```python
from build123d import *

# Parameters (mm, degrees)
BOSS_EXTRUDE1_DEPTH = 10
CUT_SWEEP1_START    = 7
CUT_SWEEP1_DEPTH    = 3


# Read off the part's stored shape, not the designer's step: Cut-Sweep1
with BuildPart() as part:
    # Sketch1 → Boss-Extrude1 (new body)
    with BuildSketch(Plane(origin=(0, 0, 0), x_dir=(1, 0, 0), z_dir=(0, 1, 0))):
        with BuildLine():
            Line((-35, 0), (35, 0))
            Line((35, 0), (35, 50))
            ThreePointArc((35, 50), (150, 165), (265, 50))
            Line((265, 50), (265, 0))
            Line((265, 0), (335, 0))
            Line((335, 0), (335, 50))
            ThreePointArc((335, 50), (150, 235), (-35, 50))
            Line((-35, 50), (-35, 0))
        make_face()
    extrude(amount=BOSS_EXTRUDE1_DEPTH)

    # Cut-Sweep1 outline → Cut-Sweep1 (cut)
    with BuildSketch(Plane(origin=(0, 0, 0), x_dir=(1, 0, 0), z_dir=(0, 1, 0)).offset(CUT_SWEEP1_START)):
        with BuildLine():
            Line((-30, 50), (-30, 0))
            Line((-30, 0), (-20, 0))
            Line((-20, 0), (-20, 50))
            ThreePointArc((-20, 50), (150, 220), (320, 50))
            Line((320, 50), (320, 0))
            Line((320, 0), (330, 0))
            Line((330, 0), (330, 50))
            ThreePointArc((330, 50), (150, 230), (-30, 50))
        make_face()
        with BuildLine():
            Line((20, 50), (20, 0))
            Line((20, 0), (30, 0))
            Line((30, 0), (30, 50))
            ThreePointArc((30, 50), (150, 170), (270, 50))
            Line((270, 50), (270, 0))
            Line((270, 0), (280, 0))
            Line((280, 0), (280, 50))
            ThreePointArc((280, 50), (150, 180), (20, 50))
        make_face()
    extrude(amount=CUT_SWEEP1_DEPTH, mode=Mode.SUBTRACT)


solid = part.part
```
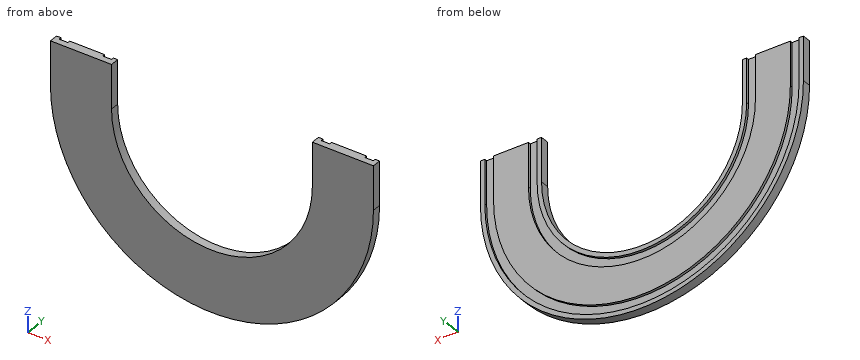
For this review, take the finished solid that the model builds, in its own axes (mm). Coordinates: 2 decimals unless noted, no trailing zeros. Write each loop counter-clockwise with the first axis right and the second up, starting at its lowest first coordinate (ties: lowest second). Pieces come first, ordered by that corner, then holes.
(1) Wall thickness on probe 1 along X at (y, z) = (1.75, -46.5); probe 2 along X at (y, z) = (7.5, -191); probe 3 along X at (y, z) = (7.5, -99.5): over which ranges is each line inside the solid? List them lowest first.
(2) Add section C-C on x = 150. Give the boundary of the cut face in (y, z).
(3) Add section A-A on z = -20. Give the boundary of the cut face in (x, y).
(4) For pin 1 Ø5 at (x, y) = (115, 8) entering from -Z; pin 2 Ø4 at (y, z) = (5, -87) entering from -X; pin 3 Ø6 at (x, y) = (99.5, 6) entering from -Z, all flat-tipped, find the tip position at first contact; note any pin that passes through.
(5) Add section D-D on z = -80.5. Give the boundary of the cut face in (x, y), then the cut area to 3 significant figures.
(6) Add section B-B on y = 4. Give the boundary of the cut face in (x, z).
Answer sheet:
1. probe 1: x = -35 to 35, 265 to 335
1. probe 2: x = 30.23 to 38.11, 55.03 to 244.97, 261.89 to 269.77
1. probe 3: x = -28.25 to -23.06, -12.63 to 29.79, 40.69 to 46.2, 253.8 to 259.31, 270.21 to 312.63, 323.06 to 328.25
2. outline: (0, -235) - (10, -235) - (10, -230) - (7, -230) - (7, -220) - (10, -220) - (10, -180) - (7, -180) - (7, -170) - (10, -170) - (10, -165) - (0, -165) - close
3. outline: (-35, 0) - (35, 0) - (35, 10) - (30, 10) - (30, 7) - (20, 7) - (20, 10) - (-20, 10) - (-20, 7) - (-30, 7) - (-30, 10) - (-35, 10) - close; (265, 0) - (335, 0) - (335, 10) - (330, 10) - (330, 7) - (320, 7) - (320, 10) - (280, 10) - (280, 7) - (270, 7) - (270, 10) - (265, 10) - close
4. pin 1: stops at z = -232.12
4. pin 2: stops at x = -31.66
4. pin 3: stops at z = -228.8
5. outline: (-32.47, 0) - (39.12, 0) - (39.12, 10) - (33.94, 10) - (33.94, 7) - (23.63, 7) - (23.63, 10) - (-17.24, 10) - (-17.24, 7) - (-27.4, 7) - (-27.4, 10) - (-32.47, 10) - close; (260.88, 0) - (332.47, 0) - (332.47, 10) - (327.4, 10) - (327.4, 7) - (317.24, 7) - (317.24, 10) - (276.37, 10) - (276.37, 7) - (266.06, 7) - (266.06, 10) - (260.88, 10) - close
5. area: 1,310 mm2
6. outline: (-35, -50) arc R185 ccw to (335, -50) - (335, 0) - (265, 0) - (265, -50) arc R115 cw to (35, -50) - (35, 0) - (-35, 0) - close
